Read the model definition and answer for the solid it produces. Units are mm, in the model's axes. Face numbers are marked on the shaded views. A direction names the side the tool comes from. Round coordinates to 2 decimals unless told otherwise and drop trailing zeros. Order: outer loops, then holes, each group sorted by start corner. A loop starts at its lowest first (then second) coordinate and runs counter-clockwise, first axis right, second up. Notation, with made-up numbers: (64, 15) - (91, 15) arc R8 ccw to (91, 20) - close; hole circle Ø9 at (-24, 69.5). An arc over 180 degrees is marked (long way). One line per question, with ' | ' between items. Start each with the question number.
1) Straight lines are drawn through the part: line 1 (X direction, y = 44.9, z = 0); line 2 (Z direction, x = -6.5, y = 42.5); line 3 (Z direction, x = -5.5, y = 24.5). For each, find the intervals that lie inside material, in ascending order. Write a range as from..to.
2) The part is cut by section D-D, the plane y = 30. Give the vertices of the cut face in (x, z) (3 decimals).
3) The part is cut by section A-A, the plane y = -1. Give the vertices of the cut face in (x, z).
4) The part is cut by section C-C, the plane z = 9.75. Give the vertices of the cut face in (x, y), plus the area to 3 significant figures.
5) For the marked faces 1, 2 and 3, determine the directions among +Z, -Z, +X, -X, +Y, -Y from which every point of the face is accessible in a straight line to the end or side of a thin tool.
6) The mould has two halves that part along Z. Classify the marked faces 4, 5, 6 and 7: pulls with the +Z half, pulls with the -Z half, needs draft (parallel to the pull), parting line crosses it, or undercut.
7) Flat-ended cylindrical pins translate along their axes: pin 1 (2.5 mm diameter, centred on y = -1.5, z = -0.5, fed in from +X); pin 2 (10 mm diameter, centred on x = 3, z = 1, fed in from +Y); pin 3 (2.5 mm diameter, centred on x = 8, z = 0, fed in from +Y); pin 4 (13.5 mm diameter, centred on x = 0.5, z = 4, fed in from -Y). Find the tip coordinate at first contact, or state that the pin passes through.
Autodesk Inventor part; units mm, degrees
ref_plane "Work Plane1" through (0, 41.5, 0) normal (0, 1, 0) x (1, 0, 0)
ref_plane "Work Plane2" through (0, 50.2, 0) normal (0, 1, 0) x (1, 0, 0)
ref_plane "YZ Plane" through (0, 0, 0) normal (1, 0, 0) x (0, 1, 0)
sketch "Sketch1" plane through (0, 0, 0) normal (0, 1, 0) x (-1, 0, 0)
  circle A0 centre (0, 0) radius 13.7
  dimension "d0" = 27.4
extrude "Extrusion1" add sketch "Sketch1" along normal blind 46.5
sketch "Sketch2" plane through (0, 46.5, 0) normal (0, 1, 0) x (1, 0, 0)
  circle A0 centre (0, 0) radius 13.7
  circle A1 centre (0, 0) radius 5
  dimension "d3" = 10
extrude "Extrusion2" add sketch "Sketch2" along normal blind 2.7 contours A1
sketch "Sketch3" plane through (0, 46.5, 0) normal (0, 1, 0) x (1, 0, 0)
  circle A0 centre (0, 0) radius 5
  circle A1 centre (0, 0) radius 5
  circle A2 centre (0, 0) radius 13.7
  circle A3 centre (0, 0) radius 13.7
  line L0 (-13.7, 0) -> (13.7, 0)
  point P0 (-8, 0)
  point P1 (8, 0)
  dimension "d6" = 16
  dimension "d7" = 5.7
  dimension "d8" = 5.7
hole "Hole1" at (-8, 46.5, 0) at (8, 46.5, 0) direction (0, -1, 0) diameter 2.1129 depth 2.8
ref_plane "Work Plane1" through (0, 41.5, 0) normal (0, 1, 0) x (1, 0, 0)
sketch "Sketch4" plane through (0, 41.5, 0) normal (0, 1, 0) x (1, 0, 0)
  circle A0 centre (0, 0) radius 14.375
  dimension "d17" = 28.75
extrude "Extrusion3" add sketch "Sketch4" against normal blind 27.7
sketch "Sketch5" plane through (0, 0, 0) normal (0, -1, 0) x (1, 0, 0)
  circle A0 centre (0, 0) radius 5
  dimension "d20" = 10
extrude "Extrusion4" add sketch "Sketch5" along normal blind 4
sketch "Sketch6" plane through (0, 0, 0) normal (0, -1, 0) x (1, 0, 0)
  circle A0 centre (0, 0) radius 5
  circle A1 centre (0, 0) radius 5
  circle A2 centre (0, 0) radius 13.7
  circle A3 centre (0, 0) radius 13.7
  line L0 (13.7, 0) -> (-13.7, 0)
  line L1 (-11.5, 1.5) -> (-12, 1.5)
  line L2 (-12, 1.5) -> (-12, -1.5)
  line L3 (-12, -1.5) -> (-11.5, -1.5)
  line L4 (-11.5, -1.5) -> (-11.5, 1.5)
  line L5 (11.5, 1.5) -> (11, 1.5)
  line L6 (11, 1.5) -> (11, -1.5)
  line L7 (11, -1.5) -> (11.5, -1.5)
  line L8 (11.5, -1.5) -> (11.5, 1.5)
  dimension "d23" = 22.5
  dimension "d24" = 0.5
  dimension "d25" = 0.5
  dimension "d26" = 11.5
  dimension "d27" = 11.5
  dimension "d28" = 3
  dimension "d29" = 3
  dimension "d30" = 1.5
  dimension "d31" = 1.5
extrude "Extrusion5" add sketch "Sketch6" along normal blind 6 contours L6 L5 L8 L0 | L0 L8 L7 L6 | L4 L3 L2 L0 | L0 L2 L1 L4
sketch "Sketch7" plane through (0, 49.2, 0) normal (0, 1, 0) x (1, 0, 0)
  circle A0 centre (0, 0) radius 1.1
  dimension "d34" = 2.2
extrude "Extrusion6" add sketch "Sketch7" along normal blind 13.5
ref_plane "Work Plane2" through (0, 50.2, 0) normal (0, 1, 0) x (1, 0, 0)
sketch "Sketch10" plane through (0, 0, 0) normal (1, 0, 0) x (0, 1, 0)
  line L0 (0, -13.7) -> (0, 13.7)
  line L1 (13.8, 13.7) -> (13.8, -13.7)
  line L2 (9, 4.6) -> (13.8, 4.6)
  line L3 (13.8, 4.6) -> (13.8, -4.6)
  line L4 (13.8, -4.6) -> (9, -4.6)
  line L5 (9, -4.6) -> (9, 4.6)
  circle A0 centre (11.4, 4.6) radius 2.4
  circle A1 centre (11.4, -4.6) radius 2.4
  line L6 (0, 0) -> (13.8, 0)
  line L7 (13.8, 13.7) -> (13.8, -13.7)
  line L8 (0, -13.7) -> (13.8, -13.7)
  point P0 (11.4, 7)
  point P1 (11.4, -7)
  point P2 (13.8, -4.6)
  dimension "d57" = 9
  dimension "d59" = 0
  dimension "d60" = 4.8
  dimension "d61" = 13.8
  dimension "d62" = 2.4
  dimension "d63" = 2.4
  dimension "d64" = 14
  dimension "d65" = 4.6
  dimension "d66" = 4.6
  dimension "d69" = 6.7
extrude "Extrusion9" cut sketch "Sketch10" along normal mid plane 31.5 contours L6 L1 A1 L5 | L5 A0 L1 L6 | A1 L4 | L4 A1 | A0 L2 | L2 A0
sketch "Sketch11" plane through (0, 46.5, 0) normal (0, 1, 0) x (1, 0, 0)
  circle A0 centre (-8, 0) radius 1.0564
  circle A1 centre (8, 0) radius 1.0564
  circle A2 centre (0, 0) radius 5
  circle A3 centre (0, 0) radius 13.7
  circle A4 centre (8, 0) radius 1.0564
  circle A5 centre (0, 0) radius 13.7
  line L0 (13.7, 0) -> (-13.7, 0)
  circle A6 centre (0, 0) radius 1.1
  circle A7 centre (0, 0) radius 9.0564
  circle A8 centre (0, 0) radius 6.9436
  circle A9 centre (8, 0) radius 1.0564
  line L1 (1.8876, -9.0564) -> (-1.9124, -9.0564)
  line L2 (-1.9124, -9.0564) -> (-1.9124, 9.0564)
  line L3 (-1.9124, 9.0564) -> (1.8876, 9.0564)
  line L4 (1.8876, 9.0564) -> (1.8876, -9.0564)
  line L5 (-0.0124, -13.7) -> (-0.0124, 13.7)
  line L6 (9.0564, -3.15) -> (-9.0564, -3.15)
  line L7 (-9.0564, -3.15) -> (-9.0564, 3.15)
  line L8 (-9.0564, 3.15) -> (9.0564, 3.15)
  line L9 (9.0564, 3.15) -> (9.0564, -3.15)
  circle A10 centre (6.8048, -4.2064) radius 1.0564
  circle A11 centre (2.9441, -7.4386) radius 1.0564
  circle A12 centre (-2.9688, -7.4287) radius 1.0564
  circle A13 centre (-6.8048, -4.2064) radius 1.0564
  circle A14 centre (-6.8048, 4.2064) radius 1.0564
  line L10 (-11.7767, 7) -> (11.7767, 7)
  circle A15 centre (-2.9688, 7.4287) radius 1.0564
  circle A16 centre (2.9441, 7.4386) radius 1.0564
  circle A17 centre (6.8048, 4.2064) radius 1.0564
  circle A18 centre (-0.0124, 10.65) radius 1.15
  point P0 (9.0564, 0)
  point P1 (7.8048, -3.2064)
  point P2 (3.3328, 8.4209)
  point P3 (2.5553, 6.4563)
  point P4 (5.9062, 3.651)
  point P5 (7.7035, 4.7619)
  point P6 (-5.9062, 3.651)
  point P7 (-2.5768, 6.4477)
  point P8 (-3.3608, 8.4097)
  point P9 (-7.7035, 4.7619)
  point P10 (-3.3608, -8.4097)
  point P11 (-2.5768, -6.4477)
  point P12 (-5.9062, -3.651)
  point P13 (-7.7035, -4.7619)
  point P14 (7.7035, -4.7619)
  point P15 (5.9062, -3.651)
  point P16 (2.5553, -6.4563)
  point P17 (3.3328, -8.4209)
  point P18 (-0.0124, 11.8)
  dimension "d78" = 2.3
  dimension "d70" = 3.8
  dimension "d71" = 1.9
  dimension "d72" = 1.9
  dimension "d73" = 6.3
  dimension "d74" = 3.15
  dimension "d75" = 3.15
  dimension "d79" = 1.9
extrude "Extrusion10" cut sketch "Sketch11" against normal blind 30 contours A14 A7 L10 A15 A8 | A14 | A8 A12 A7 A13 | A13 | A15 L10 | A12 | A7 A15 L10 | A15 L10 | A18 L5 | L5 A18 | L10 A16 A7 | A7 A17 A8 A16 L10 | A11 A8 A10 A7 | A11 | A17 | A16 L10 | A16 L10 | A10
equation "\"d26\" = d27"
equation "\"d30\" = d31"
equation "\"d65\" = d66"
equation "\"d71\" = d72"
equation "\"d74\" = d75"
equation "\"d41\" = d42"
properties part number "rs390" material "Steel, Mild"
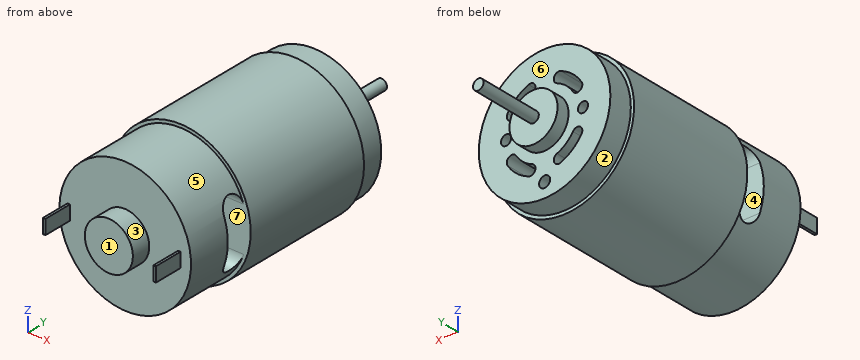
Values:
1) line 1: x = -13.7..-9.06, -6.94..6.94, 9.06..13.7 | line 2: z = -12.06..-6.31, -3.19..3.19, 6.31..12.06 | line 3: z = -13.28..-7.2, -4.24..4.24, 7.2..13.28
2) outline: circle Ø28.75 at (0, 0); hole (-7.703, -4.762) arc R9.056 ccw to (-3.361, -8.41) arc R1.056 ccw to (-2.577, -6.448) arc R6.944 cw to (-5.906, -3.651) arc R1.056 ccw to start; hole (-7.703, 4.762) arc R1.056 ccw to (-5.906, 3.651) arc R6.944 cw to (-2.577, 6.448) arc R1.056 ccw to (-3.361, 8.41) arc R9.056 ccw to start; hole circle Ø2.3 at (-0.012, -10.65); hole (2.555, -6.456) arc R1.056 ccw to (3.333, -8.421) arc R9.056 ccw to (7.703, -4.762) arc R1.056 ccw to (5.906, -3.651) arc R6.944 cw to start; hole (2.555, 6.456) arc R6.944 cw to (5.906, 3.651) arc R1.056 ccw to (7.703, 4.762) arc R9.056 ccw to (3.333, 8.421) arc R1.056 ccw to start
3) outline: (-12, -1.5) - (-11.5, -1.5) - (-11.5, 1.5) - (-12, 1.5) - close; circle Ø10 at (0, 0); (11, -1.5) - (11.5, -1.5) - (11.5, 1.5) - (11, 1.5) - close
4) outline: (-10.56, 13.8) - (-9.62, 13.8) - (-9.62, 0) - (9.62, 0) - (9.62, 13.8) - (10.56, 13.8) - (10.56, 41.5) - (9.62, 41.5) - (9.62, 46.5) - (-9.62, 46.5) - (-9.62, 41.5) - (-10.56, 41.5) - close | area: 947 mm^2
5) face 1: +Z, -Z, -Y | face 2: +Y | face 3: -Y
6) face 4: undercut | face 5: parting line crosses it | face 6: needs draft | face 7: undercut
7) pin 1: stops at x = 11.5 | pin 2: stops at y = 62.7 | pin 3: stops at y = 46.5 | pin 4: stops at y = -4
